Input: dimensioned drawing with shaded views. Units: mm. Origin: part minimum x, y, z. Round coordinates to 2 decimals unless told otherwise and drop trailing zeros. Loops run counter-clockwise (first coordinate to the right, second up) from the corner with the lowest first, then second, coordinate; pieces in that order, holes last. Notation, with made-up numbers: M 6.5,52.5 L 59.5,52.5 A24 ccw 59.5,70.5 Z; hole C -23,40 d11. An arc over 180 degrees is marked long. Put each result on its own line as item: value. Start each with the question number.
1) Pin query (flat end, axial travel): pin 1 (3 mm diameter, centred on x = 35.64, z = 4.44, fed in from -Y). Return the tip coordinate at first contact, or that it passes through.
2) Section B-B on x = 36.5. Output: boundary loops of the cut face in (y, z) (1 decimal).
3) Line query: probe 1 along X at (y, z) = (0.3, 55.5); probe 2 along Z at (x, y) = (35.5, 2); probe 3 along X at (y, z) = (1.1, 20.5). Output: solid intervals per line, ascending.
4) Section A-A on y = 1.9. State how many separate pieces and enclosed holes the cut face has, plus the area to 3 significant figures.
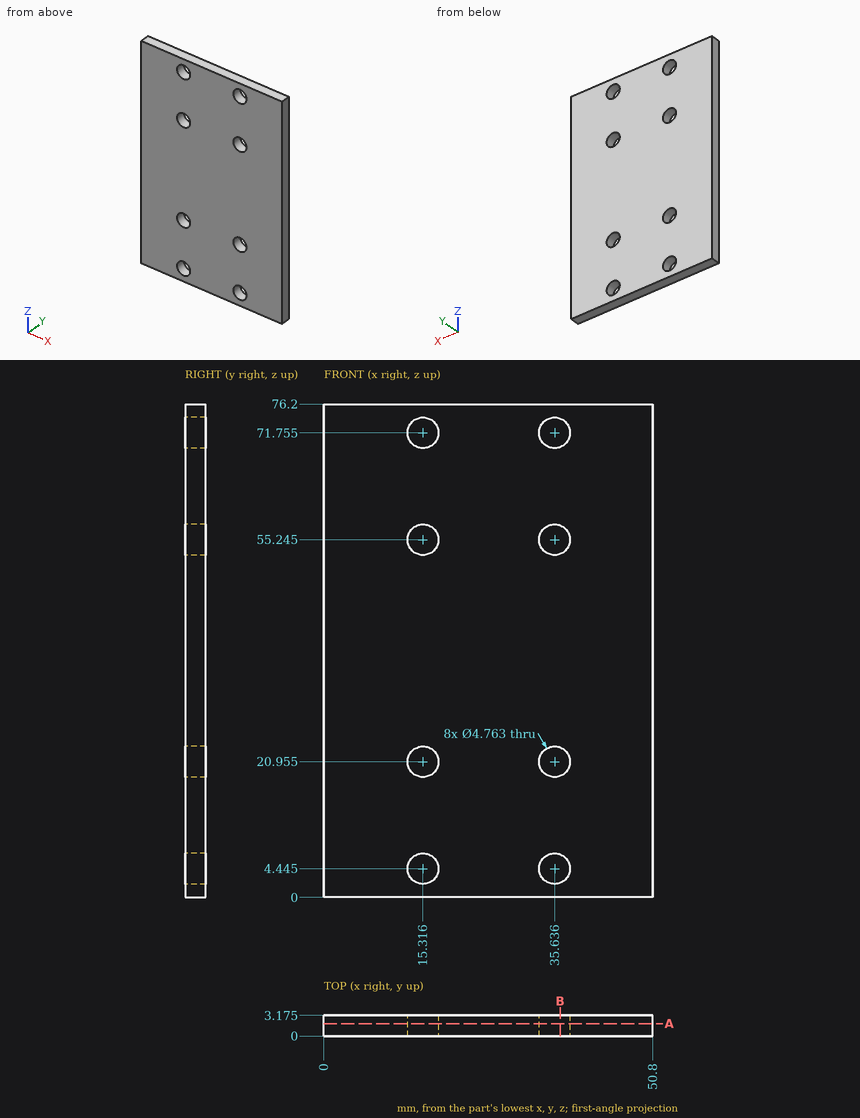
Geometry results:
1. pin 1: passes through
2. outline: M 0,0 L 3.2,0 L 3.2,2.2 L 0,2.2 Z; M 0,6.7 L 3.2,6.7 L 3.2,18.7 L 0,18.7 Z; M 0,23.2 L 3.2,23.2 L 3.2,53 L 0,53 Z; M 0,57.5 L 3.2,57.5 L 3.2,69.5 L 0,69.5 Z; M 0,74 L 3.2,74 L 3.2,76.2 L 0,76.2 Z
3. probe 1: x = 0 to 12.95, 17.68 to 33.27, 38 to 50.8
3. probe 2: z = 0 to 2.07, 6.82 to 18.58, 23.33 to 52.87, 57.62 to 69.38, 74.13 to 76.2
3. probe 3: x = 0 to 12.98, 17.65 to 33.3, 37.97 to 50.8
4. separate pieces: 1
4. enclosed holes: 8
4. area: 3,730 mm²
